Geometry: final body of the model. Coordinates: model frame, mm. A direction names the side the tool comes from. Give positions to 0.01 mm unless a question says otherwise; leave off trailing zeros. Write each loop counter-clockwise with the first axis right and the second up, starting at its lowest first coordinate (ties: lowest second). Pieces come first, ordered by that corner, then holes. Notation, with made-up numbers: (23.25, 10) -> (81.25, 10) arc R19 cw to (81.25, 42) -> close; hole circle Ø11 at (8, 78.25). An arc over 180 degrees is marked (long way). Answer as a JSON object with one key per item and string values. Group by question number.
(1) Section query D-D on x = 2. Output: boundary loops of the cut face in (y, z), plus the area to 3 significant figures.
(2) Contact query for flat-ended pins moving along their axis: pin 1 Ø8 at (x, y) = (9, 8.5) entering from -Z; pin 2 Ø8 at (x, y) = (11, 7) entering from +Z; pin 3 Ø1 at (x, y) = (12.5, -7.5) entering from +Z. Output: stop coordinate, or through.
(3) Draft query along Y for faces 3 (the face through (10.97, 8.23, 2.59)), 4 (the face through (18, -3, 0)), 5 (the face through (9.126, -2.636, 0.585)). Return one class per face: +Y half, -Y half, draft (parallel to the pull), parting line (faces both ways), or undercut.
(4) Material intervals for probe 1 along X at (y, z) = (-7, -6.5); probe 2 along X at (y, z) = (-0.5, -11); probe 3 along Y at (x, z) = (5.75, 0), sorted ascending.
(5) Section query A-A on z = 0. Output: boundary loops of the cut face in (x, y).
(6) Section query C-C on x = 14. Output: boundary loops of the cut face in (y, z), plus the area to 3 significant figures.
(7) Set-up query: faces 1 (the face through (0, -3, 0)), 2 (the face through (7.14, -8.51, 0.37)). Return all of +Z, -Z, +X, -X, +Y, -Y with unobstructed straight access to the full face (end or side cutting, diameter ignored); none if empty.
from build123d import *

# Parameters (mm, degrees)
SKETCH1_R           = 17.5
BOSS_EXTRUDE1_DEPTH = 18
SKETCH2_R           = 2.7
CUT_EXTRUDE1_DEPTH  = 18


with BuildPart() as part:
    # Sketch1 → Boss-Extrude1 (new body)
    with BuildSketch(Plane(origin=(0, 0, 0), x_dir=(0, 0, -1), z_dir=(1, 0, 0))):
        Circle(SKETCH1_R)
    extrude(amount=BOSS_EXTRUDE1_DEPTH)

    # Sketch2 → Cut-Extrude1 (cut)
    with BuildSketch(Plane(origin=(18, 0, 0), x_dir=(0, 0, -1), z_dir=(1, 0, 0))):
        Circle(SKETCH2_R)
    extrude(amount=-CUT_EXTRUDE1_DEPTH, mode=Mode.SUBTRACT)

    # Sketch3 → Cut-Revolve1 (revolve, cut)
    with BuildSketch(Plane.XY):
        with BuildLine():
            Line((10.5, 8.155563792), (24.900813008, 22.5563768))
            Line((24.900813008, 22.5563768), (-6.900813008, 22.5563768))
            Line((-6.900813008, 22.5563768), (7.5, 8.155563792))
            ThreePointArc((7.5, 8.155563792), (9, 7.534243448), (10.5, 8.155563792))
        make_face()
    revolve(axis=Axis((0, 0, 0), (1, 0, 0)), mode=Mode.SUBTRACT)


solid = part.part
Answer list:
{
 "1": {"outline": "circle Ø27.31 at (0, 0); hole circle Ø5.4 at (0, 0)", "area": "563 mm2"},
 "2": {"pin 1": "z = -7.76", "pin 2": "z = 11.08", "pin 3": "z = 7.72"},
 "3": {"face 3": "parting line", "face 4": "draft", "face 5": "undercut"},
 "4": {"probe 1": "0 to 6.1, 11.9 to 18", "probe 2": "0 to 4.64, 13.36 to 18", "probe 3": "-9.91 to -2.7, 2.7 to 9.91"},
 "5": {"outline": "(0, -15.66) -> (7.5, -8.16) arc R2.12 cw to (10.5, -8.16) -> (18, -15.66) -> (18, -2.7) -> (0, -2.7) -> close; (0, 2.7) -> (18, 2.7) -> (18, 15.66) -> (10.5, 8.16) arc R2.12 cw to (7.5, 8.16) -> (0, 15.66) -> close"},
 "6": {"outline": "circle Ø23.31 at (0, 0); hole circle Ø5.4 at (0, 0)", "area": "404 mm2"},
 "7": {"face 1": "+Z, -Z, -X, +Y, -Y", "face 2": "none"}
}
